Verification items for this drawing (mm, ordinates from the low corner). Coordinates: 2 decimals unless noted, no trailing zeros. Write each loop counter-clockwise with the first axis right and the second up, starting at its lowest first coordinate (ties: lowest second). Pieces come first, ordered by that corner, then holes. Notation, with made-up numbers: (-12, -2.5) -> (36, -2.5) arc R11 cw to (36, 7.5) -> close; hole circle Ø3 at (6.5, -14.5). An arc over 180 degrees is marked (long way). Answer as CSV lines item,"result".
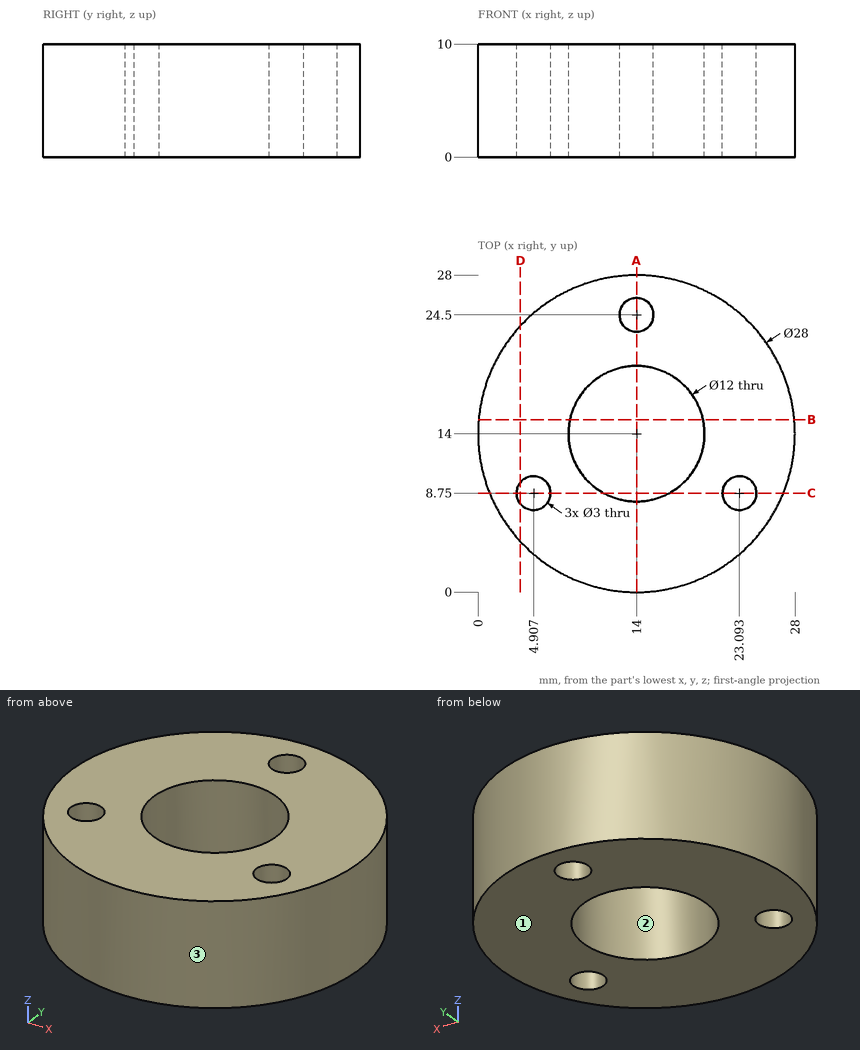
Item 1: Cross-section at B-B, the plane y = 15.25. Record the cut outline in (x, z).
Responses:
outline,"(0.06, 0) -> (8.13, 0) -> (8.13, 10) -> (0.06, 10) -> close; (19.87, 0) -> (27.94, 0) -> (27.94, 10) -> (19.87, 10) -> close"
Item 2: Cross-section at A-A, the plane x = 14. Record the cut outline in (y, z), plus the area to 3 significant figures.
Responses:
outline,"(0, 0) -> (8, 0) -> (8, 10) -> (0, 10) -> close; (20, 0) -> (23, 0) -> (23, 10) -> (20, 10) -> close; (26, 0) -> (28, 0) -> (28, 10) -> (26, 10) -> close"
area,"130 mm2"
Item 3: Cross-section at D-D, the plane x = 3.75. Record the cut outline in (y, z) (1 decimal), plus the area to 3 significant figures.
Responses:
outline,"(4.5, 0) -> (7.8, 0) -> (7.8, 10) -> (4.5, 10) -> close; (9.7, 0) -> (23.5, 0) -> (23.5, 10) -> (9.7, 10) -> close"
area,"172 mm2"
Item 4: Cross-section at C-C, the plane y = 8.75. Record the cut outline in (x, z) (1 decimal).
Responses:
outline,"(1, 0) -> (3.4, 0) -> (3.4, 10) -> (1, 10) -> close; (6.4, 0) -> (11.1, 0) -> (11.1, 10) -> (6.4, 10) -> close; (16.9, 0) -> (21.6, 0) -> (21.6, 10) -> (16.9, 10) -> close; (24.6, 0) -> (27, 0) -> (27, 10) -> (24.6, 10) -> close"
Item 5: Release check for a two-part mould opening along Y. For the marked faces 1, 2 and 3 record: +Y half, -Y half, draft (parallel to the pull), parting line (faces both ways), or undercut.
Responses:
face 1,"draft"
face 2,"undercut"
face 3,"parting line"
Item 6: Depth check by flat-ended pin: pin 1 Ø1 at (x, z) = (15, 6.5) entering from -Y; pin 2 Ø1.5 at (y, z) = (18.5, 3.5) entering from +X; pin 3 Ø1.5 at (x, z) = (4, 1.5) entering from +Y; pin 4 Ø2.5 at (x, y) = (23.09, 8.75) entering from +Z. Enter the tip coordinate at first touch or a pass-through.
Responses:
pin 1,"stops at y = 0.01"
pin 2,"stops at x = 27.49"
pin 3,"stops at y = 24.51"
pin 4,"passes through"
Item 7: Thickness scan on probe 1 along Y at (x, z) = (14, 7.5); probe 2 along X at (y, z) = (7.75, 6.5) (1 decimal); probe 3 along Y at (x, z) = (23, 7) (1 decimal). Record the ranges inside material, lowest first.
Responses:
probe 1,"y = 0 to 8, 20 to 23, 26 to 28"
probe 2,"x = 1.5 to 3.8, 6 to 22, 24.2 to 26.5"
probe 3,"y = 3.3 to 7.3, 10.2 to 24.7"
